Verification items for the finished model (mm, model axes). Round coordinates to 2 decimals unless told otherwise and drop trailing zeros. Loops run counter-clockwise (first coordinate to the right, second up) from the corner with the lowest first, then second, coordinate; pieces in that order, holes last. Notation, with made-up numbers: M 44.25,76.5 L 56.25,76.5 A13 ccw 56.25,94.5 Z; hole C 70,14 d1. An arc over 180 degrees is marked long. Write item = value, one per line. Start each with the question number.
from build123d import *

# Parameters (mm, degrees)
F1_DEPTH = 10


with BuildPart() as f1:
    # F0 (on Front) → F1 (new body)
    with BuildSketch(Plane.XZ):
        Polygon((76, 172.676718), (0, 241.080747), (-76, 172.676718), (-76, -317.323282), (0, -248.919253), (76, -317.323282), align=None)
        Polygon((-56, -151.845365), (0, -108.919253), (56, -151.845365), (56, -221.845365), (0, -178.919253), (-56, -221.845365), align=None, mode=Mode.SUBTRACT)
        Polygon((-56, -11.845365), (0, 31.080747), (56, -11.845365), (56, -81.845365), (0, -38.919253), (-56, -81.845365), align=None, mode=Mode.SUBTRACT)
        Polygon((-56, 128.102943), (0, 167.964432), (56, 128.102943), (56, 61.219258), (0, 101.080747), (-56, 61.219258), align=None, mode=Mode.SUBTRACT)
    extrude(amount=F1_DEPTH)


solid = f1.part
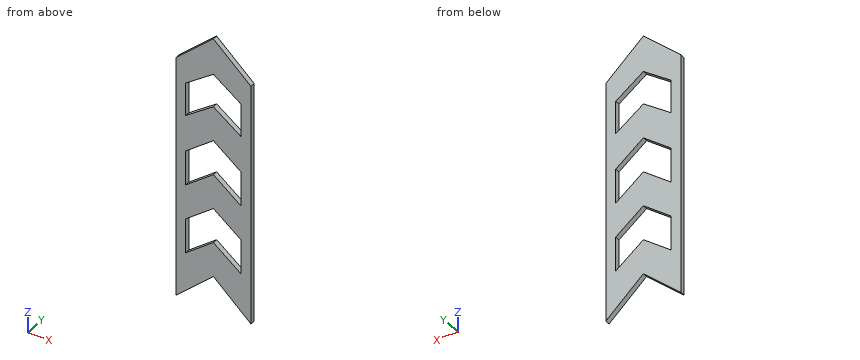
1. Section check D-D, the plane x = -67. Enter the section's corners in (y, z), and give its area (3 significant figures).
2. Gauge pin test, flat ends, axial feed: P1, Ø6, axis at x = -41, y = -5, coming from the +Z side; P2, Ø1, axis at x = 8.5, y = -2.5, coming from the -Z side; P3, Ø3, axis at x = 53, y = -3, coming from the -Z side. Record the tip position at first contact, or that the pin passes through.
3. Section check B-B, the plane z = -216.5. Enter the section's corners in (x, y).
4. Section check C-C, the plane x = -28. Enter the section's corners in (y, z), and give its area (3 significant figures).
5. Thickness scan on line 1 (Z direction, x = 55, y = -3); line 2 (Z direction, x = 14, y = -5.75); line 3 (X direction, y = -2.5, z = -164). Record the ranges inside material, lowest first.
6. Section check A-A, the plane y = -5.25. Enter the section's corners in (x, z).
Computed values:
q1.outline = M -10,-309.22 L 0,-309.22 L 0,180.78 L -10,180.78 Z
q1.area = 4,900 mm2
q2.P1 = 206.88
q2.P2 = -257.02
q2.P3 = -297.97
q3.outline = M -76,-10 L -56,-10 L -56,0 L -76,0 Z; M -49.03,-10 L 49.03,-10 L 49.03,0 L -49.03,0 Z; M 56,-10 L 76,-10 L 76,0 L 56,0 Z
q4.outline = M -10,-274.12 L 0,-274.12 L 0,-200.38 L -10,-200.38 Z; M -10,-130.38 L 0,-130.38 L 0,-60.38 L -10,-60.38 Z; M -10,9.62 L 0,9.62 L 0,81.15 L -10,81.15 Z; M -10,148.03 L 0,148.03 L 0,215.88 L -10,215.88 Z
q4.area = 2,830 mm2
q5.line_1 = -298.42 to -221.08, -151.08 to -81.08, -11.08 to 61.93, 128.81 to 191.58
q5.line_2 = -261.52 to -189.65, -119.65 to -49.65, 20.35 to 91.12, 158 to 228.48
q5.line_3 = -76 to -56, 56 to 76
q6.outline = M -76,-317.32 L 0,-248.92 L 76,-317.32 L 76,172.68 L 0,241.08 L -76,172.68 Z; hole M -56,-221.85 L 0,-178.92 L 56,-221.85 L 56,-151.85 L 0,-108.92 L -56,-151.85 Z; hole M -56,-81.85 L 0,-38.92 L 56,-81.85 L 56,-11.85 L 0,31.08 L -56,-11.85 Z; hole M -56,61.22 L 0,101.08 L 56,61.22 L 56,128.1 L 0,167.96 L -56,128.1 Z
